Geometry: final body of the model. Coordinates: model frame, mm. A direction names the side the tool comes from. Give positions to 0.01 mm unless a question says otherwise; leave off trailing zeros. Write each loop counter-clockwise with the first axis right and the second up, starting at its lowest first coordinate (ties: lowest second). Pieces come first, ordered by that corner, then holes.
```python
from build123d import *

# Parameters (mm, degrees)
SKETCH_1_W          = 5
SKETCH_1_H          = 7
EXTRUDE_1_DEPTH     = 11
SKETCH_3_R          = 1.575
CUT_EXTRUDE_1_DEPTH = 7
SKETCH_4_R          = 1.55
CUT_EXTRUDE_2_DEPTH = 7
SKETCH_5_W          = 5
SKETCH_5_H          = 2.6
CUT_EXTRUDE_3_DEPTH = 5


with BuildPart() as part:
    # Эскиз1 → Бобышка-Вытянуть1 (new body)
    with BuildSketch(Plane(origin=(0, 0, 0), x_dir=(1, 0, 0), z_dir=(0, 1, 0))):
        Rectangle(SKETCH_1_W, SKETCH_1_H)
    extrude(amount=EXTRUDE_1_DEPTH)

    # Эскиз3 → Вырез-Вытянуть1 (cut)
    with BuildSketch(Plane(origin=(0, 11, 0), x_dir=(1, 0, 0), z_dir=(0, 1, 0))):
        with Locations(Location((0, -1.3, 0), (0, 0, 270))):
            Circle(SKETCH_3_R)
    extrude(amount=-CUT_EXTRUDE_1_DEPTH, mode=Mode.SUBTRACT)

    # Эскиз4 → Вырез-Вытянуть2 (cut)
    with BuildSketch(Plane(origin=(0, 0, -3.5), x_dir=(-1, 0, 0), z_dir=(0, 0, -1))):
        with Locations((0, 2.1)):
            Circle(SKETCH_4_R)
    extrude(amount=-CUT_EXTRUDE_2_DEPTH, mode=Mode.SUBTRACT)

    # Эскиз5 → Вырез-Вытянуть3 (cut)
    with BuildSketch(Plane(origin=(0, 11, 0), x_dir=(1, 0, 0), z_dir=(0, 1, 0))):
        with Locations((0, 2.2)):
            Rectangle(SKETCH_5_W, SKETCH_5_H)
    extrude(amount=-CUT_EXTRUDE_3_DEPTH, mode=Mode.SUBTRACT)


solid = part.part
```
Item 1: Pin query (flat end, axial travel): pin 1 Ø1.5 at (x, y) = (-0.5, 8) entering from -Z; pin 2 Ø0.9 at (x, z) = (0.5, 2) entering from +Y; pin 3 Ø2 at (x, z) = (0, -3) entering from +Y. Return the tip coordinate at first contact, or that it passes through.
Found:
pin 1: stops at z = -0.9
pin 2: stops at y = 4
pin 3: stops at y = 6
Item 2: Section B-B, the plane x = 0. Return the cut outline in (y, z) (3 decimals), plus the area to 4 significant figures.
Found:
outline: (0, -3.5) - (0.55, -3.5) - (0.55, 3.5) - (0, 3.5) - close; (3.65, -3.5) - (6, -3.5) - (6, -0.9) - (11, -0.9) - (11, -0.275) - (4, -0.275) - (4, 2.875) - (11, 2.875) - (11, 3.5) - (3.65, 3.5) - close
area: 20.25 mm2
Item 3: Line query: L1, parallel to X at y = 6, z = 1.3 (3 decimals); L2, parallel to Y at x = 0, z = 1.75; L3, parallel to Y at x = 0, z = -1. Output: solid intervals per line, ascending.
Found:
L1: x = -2.5 to -1.575, 1.575 to 2.5
L2: y = 0 to 0.55, 3.65 to 4
L3: y = 0 to 0.55, 3.65 to 6
Item 4: Section C-C, the plane y = 9.75. Return the cut outline in (x, z) (3 decimals), plus the area to 3 significant figures.
Found:
outline: (-2.5, -0.9) - (2.5, -0.9) - (2.5, 3.5) - (-2.5, 3.5) - close; hole circle Ø3.15 at (0, 1.3)
area: 14.2 mm2
Item 5: Section D-D, the plane z = 1.3. Return the cut outline in (x, y) (3 decimals), plus the area to 3 significant figures.
Found:
outline: (-2.5, 0) - (2.5, 0) - (2.5, 11) - (1.575, 11) - (1.575, 4) - (-1.575, 4) - (-1.575, 11) - (-2.5, 11) - close; hole circle Ø3.1 at (0, 2.1)
area: 25.4 mm2
Item 6: Reachability of faces 1 (the face through (0, 9, -0.9)), 2 (the face through (-2, 11, 1)), 3 (the face through (0, 4, 1)) from +Z, -Z, +X, -X, +Y, -Y: full face, straight path, thin tool, end or side. Return the list, or none.
Found:
face 1: -Z, +X, -X, +Y
face 2: +Z, -Z, +X, -X, +Y
face 3: +Y
Item 7: Pull-direction query (X, two-part tool) for faces 4 (the face through (0.473, 7.549, 2.802)), 5 (the face through (0.202, 3.637, -0.049)), 6 (the face through (0, 5, 3.5)), 7 (the face through (2.5, 5, 1)); classes: +X half, -X half, draft (parallel to the pull), parting line (faces both ways), or undercut.
Found:
face 4: undercut
face 5: undercut
face 6: draft
face 7: +X half
Item 8: Section A-A, the plane y = 2.1. Return the cut outline in (x, z).
Found:
outline: (-2.5, -3.5) - (-1.55, -3.5) - (-1.55, 3.5) - (-2.5, 3.5) - close; (1.55, -3.5) - (2.5, -3.5) - (2.5, 3.5) - (1.55, 3.5) - close
